Read the model definition and answer for the solid it produces. Units are mm, in the model's axes. Face numbers are marked on the shaded views. A direction names the side the tool comes from. Round coordinates to 2 decimals unless told otherwise and drop trailing zeros. Loops run counter-clockwise (first coordinate to the right, second up) from the corner with the lowest first, then second, coordinate; pieces in that order, holes last. Notation, with made-up numbers: (-28, -0.5) -> (13, -0.5) arc R23 ccw to (13, 34.5) -> close; hole circle Ø6 at (-4, 79). An arc over 180 degrees is marked (long way). Put each result on its own line as item: value.
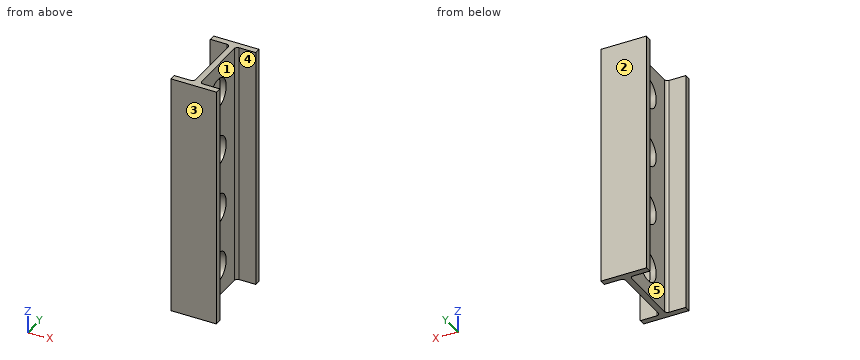
Autodesk Fusion 360 part; units mm, degrees
sketch "Sketch1" plane through (0, 0, 0) normal (0, 0, 1) x (1, 0, 0)
  line L0 (0, 0) -> (97.8805, 0) construction
  line L1 (0.5, 0) -> (0.5, 5)
  arc A0 (1, 5.5) -> (0.5, 5) centre (1, 5) ccw
  line L2 (1, 5.5) -> (3.75, 5.5)
  line L3 (3.75, 5.5) -> (3.75, 6.5)
  line L4 (3.75, 6.5) -> (0, 6.5)
  line L5 (0, 0) -> (0, 6.5) construction
  line L6 (-3.75, 6.5) -> (0, 6.5)
  line L7 (-3.75, 5.5) -> (-3.75, 6.5)
  line L8 (-1, 5.5) -> (-3.75, 5.5)
  arc A1 (-0.5, 5) -> (-1, 5.5) centre (-1, 5) ccw
  line L9 (-0.5, 0) -> (-0.5, 5)
  line L10 (-3.75, -6.5) -> (0, -6.5)
  line L11 (-3.75, -5.5) -> (-3.75, -6.5)
  line L12 (-1, -5.5) -> (-3.75, -5.5)
  arc A2 (-1, -5.5) -> (-0.5, -5) centre (-1, -5) ccw
  line L13 (-0.5, 0) -> (-0.5, -5)
  line L14 (0.5, 0) -> (0.5, -5)
  arc A3 (0.5, -5) -> (1, -5.5) centre (1, -5) ccw
  line L15 (1, -5.5) -> (3.75, -5.5)
  line L16 (3.75, -5.5) -> (3.75, -6.5)
  line L17 (3.75, -6.5) -> (0, -6.5)
  dimension "d1" = 0.5
  dimension "d2" = 0.5
  dimension "d3" = 1
  dimension "d4" = 5.5
  dimension "d5" = 3.25
extrude "Extrude1" add sketch "Sketch1" along normal blind 40
sketch "Sketch2" plane through (0.5, 0, 0) normal (1, 0, 0) x (0, 0, -1)
  line L0 (0, -5) -> (0, 5)
  line L1 (0, 5) -> (-40, 5)
  line L2 (-40, 5) -> (-40, -5)
  line L3 (-40, -5) -> (0, -5)
  line L4 (0, 0) -> (-40, 0) construction
  circle A0 centre (-35, 0) radius 2.5
  circle A1 centre (-25, 0) radius 2.5
  circle A2 centre (-15, 0) radius 2.5
  circle A3 centre (-5, 0) radius 2.5
  point P0 (-5, 0)
  point P1 (-25, 0)
  point P2 (-35, 0)
  point P3 (-15, 0)
  dimension "d8" = 5
  dimension "d9" = 15
  dimension "d10" = 25
  dimension "d11" = 35
  dimension "d12" = 5
  dimension "d13" = 5
  dimension "d14" = 5
  dimension "d15" = 5
extrude "Extrude2" cut sketch "Sketch2" against normal through all contours A0 | A1 | A2 | A3
Item 1: Which of the six approach directions +Z, -Z, +X, -X, +Y, -Y give full straight-line access (tool end or side, diameter ignored) to the marked faces 4 and 5?
Derived:
face 4: +Z, -Z, +X
face 5: +Z, -Z, -X
Item 2: The part is cut by section D-D (z = 15.5). Determine the outline of the cut face in (x, y), then the cut area to 3 significant figures.
Derived:
outline: (-3.75, -6.5) -> (3.75, -6.5) -> (3.75, -5.5) -> (1, -5.5) arc R0.5 cw to (0.5, -5) -> (0.5, -2.45) -> (-0.5, -2.45) -> (-0.5, -5) arc R0.5 cw to (-1, -5.5) -> (-3.75, -5.5) -> close; (-3.75, 5.5) -> (-1, 5.5) arc R0.5 cw to (-0.5, 5) -> (-0.5, 2.45) -> (0.5, 2.45) -> (0.5, 5) arc R0.5 cw to (1, 5.5) -> (3.75, 5.5) -> (3.75, 6.5) -> (-3.75, 6.5) -> close
area: 21.3 mm^2
Item 3: For a pull along Y with two mould halves and no side action, classify the marked faces 1, 2 and 3 as pulls with the +Y half, pulls with the -Y half, needs draft (parallel to the pull), parting line crosses it, or undercut.
Derived:
face 1: undercut
face 2: pulls with the +Y half
face 3: pulls with the -Y half
Item 4: Find the intervals of material crossed by line 1 along Z through (x, y) = (0, 0); line 2 along Y through (x, z) = (0.3, 5); line 3 along Y through (x, z) = (-1.25, 6), in increasing order.
Derived:
line 1: z = 0 to 2.5, 7.5 to 12.5, 17.5 to 22.5, 27.5 to 32.5, 37.5 to 40
line 2: y = -6.5 to -2.5, 2.5 to 6.5
line 3: y = -6.5 to -5.5, 5.5 to 6.5
Item 5: The part is cut by section C-C (y = 2). Determine the outline of the cut face in (x, z).
Derived:
outline: (-0.5, 0) -> (0.5, 0) -> (0.5, 3.5) -> (-0.5, 3.5) -> close; (-0.5, 6.5) -> (0.5, 6.5) -> (0.5, 13.5) -> (-0.5, 13.5) -> close; (-0.5, 16.5) -> (0.5, 16.5) -> (0.5, 23.5) -> (-0.5, 23.5) -> close; (-0.5, 26.5) -> (0.5, 26.5) -> (0.5, 33.5) -> (-0.5, 33.5) -> close; (-0.5, 36.5) -> (0.5, 36.5) -> (0.5, 40) -> (-0.5, 40) -> close
Item 6: The part is cut by section B-B (z = 3). Determine the outline of the cut face in (x, y).
Derived:
outline: (-3.75, -6.5) -> (3.75, -6.5) -> (3.75, -5.5) -> (1, -5.5) arc R0.5 cw to (0.5, -5) -> (0.5, -1.5) -> (-0.5, -1.5) -> (-0.5, -5) arc R0.5 cw to (-1, -5.5) -> (-3.75, -5.5) -> close; (-3.75, 5.5) -> (-1, 5.5) arc R0.5 cw to (-0.5, 5) -> (-0.5, 1.5) -> (0.5, 1.5) -> (0.5, 5) arc R0.5 cw to (1, 5.5) -> (3.75, 5.5) -> (3.75, 6.5) -> (-3.75, 6.5) -> close
Item 7: Flat-ended cylindrical pins translate along their axes: pin 1 Ø6 at (y, z) = (0, 5) entering from -X; pin 2 Ø1 at (y, z) = (-3, 18.5) entering from +X; pin 3 Ø2 at (y, z) = (1, 6) entering from +X. Find the tip coordinate at first contact, or state that the pin passes through.
Derived:
pin 1: stops at x = -0.5
pin 2: stops at x = 0.5
pin 3: passes through
Item 8: The part is cut by section A-A (x = -2.25). Determine the outline of the cut face in (y, z), then the cut area to 3 significant figures.
Derived:
outline: (-6.5, 0) -> (-5.5, 0) -> (-5.5, 40) -> (-6.5, 40) -> close; (5.5, 0) -> (6.5, 0) -> (6.5, 40) -> (5.5, 40) -> close
area: 80.0 mm^2
